Autodesk Inventor part; units mm, degrees
ref_plane "YZ Plane" through (0, 0, 0) normal (1, 0, 0) x (0, 1, 0)
ref_plane "XZ Plane" through (0, 0, 0) normal (0, 1, 0) x (-1, 0, 0)
ref_plane "XY Plane" through (0, 0, 0) normal (0, 0, 1) x (1, 0, 0)
sketch "Sketch1" plane through (0, 0, 0) normal (0, 1, 0) x (-1, 0, 0)
  line L0 (0, 0) -> (50, 0)
  line L1 (50, 0) -> (50, 460)
  line L2 (50, 460) -> (0, 460)
  line L3 (0, 460) -> (0, 0)
  circle A0 centre (25, 415) radius 12
  circle A1 centre (25, 45) radius 12
  circle A2 centre (25, 450) radius 5
  circle A3 centre (25, 10) radius 5
  line L4 (50, 280) -> (0, 280)
  line L5 (0, 280) -> (0, 180)
  line L6 (0, 180) -> (50, 180)
  line L7 (50, 180) -> (50, 280)
  circle A4 centre (25, 170) radius 5
  circle A5 centre (25, 290) radius 5
  circle A6 centre (25, 230) radius 5
  dimension "d0" = 50
  dimension "d1" = 460
  dimension "d2" = 45
  dimension "d3" = 24
  dimension "d4" = 45
  dimension "d5" = 10
  dimension "d6" = 10
  dimension "d7" = 10
  dimension "d8" = 10
  dimension "d9" = 25
  dimension "d10" = 25
  dimension "d11" = 25
  dimension "d12" = 25
  dimension "d15" = 50
  dimension "d16" = 100
  dimension "d17" = 180
  dimension "d18" = 10
  dimension "d20" = 10
  dimension "d21" = 10
  dimension "d22" = 25
  dimension "d23" = 25
  dimension "d24" = 10
  dimension "d27" = 10
  dimension "d28" = 25
  dimension "d29" = 50
extrude "Plate3" add sketch "Sketch1" along normal blind 2
fillet "Fillet3" radius 15 4 edges at (0, 1, 460) (-50, 1, 460) (0, 1, 0) (-50, 1, 0)
sketch "Sketch3" plane through (0, 2, 0) normal (0, 1, 0) x (1, 0, 0)
  circle A0 centre (-25, -105) radius 12.5
  circle A1 centre (-25, -45) radius 12
  circle A2 centre (-25, -355) radius 12.5
  circle A3 centre (-25, -415) radius 12
  point P0 (0, 0)
  dimension "d36" = 25
  dimension "d37" = 60
  dimension "d38" = 25
  dimension "d42" = 60
extrude "Extrusion1" cut sketch "Sketch3" against normal blind 10 contours A0 | A2
equation "\"d30\" = Thickness"
equation "\"BendRadius\" = Thickness"
equation "\"BendReliefWidth\" = Thickness"
equation "\"BendReliefDepth\" = 0.5 * Thickness"
equation "\"CornerReliefSize\" = 4 * Thickness"
equation "\"MinimumRemnant\" = 2 * Thickness"
equation "\"TransitionRadius\" = BendRadius"
equation "\"JacobiRadiusSize\" = BendRadius"
equation "\"GapSize\" = Thickness"
properties part number "chassisPart1"
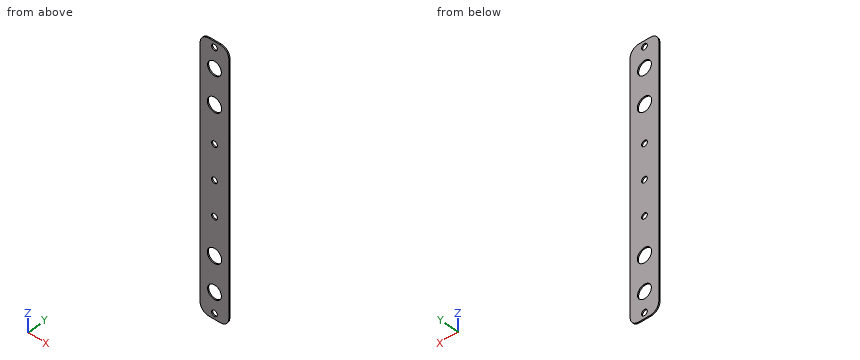
Geometry check sheet. Reference: the model listing, model coordinates, mm. Give positions to 0.01 mm unless a question says otherwise; leave off trailing zeros. Loops run counter-clockwise (first coordinate to the right, second up) from the corner with the lowest first, then second, coordinate; pieces in that order, holes last. Notation, with made-up numbers: M 64.25,-35.5 L 114.25,-35.5 A16 ccw 114.25,-21.5 Z; hole C -32,26 d4. An arc over 180 degrees is marked long. Answer as a JSON object with one key per item and string values. Group by question number.
Item 1: Material ranges on L1, parallel to Z at x = -17.5, y = 0.5; L2, parallel to Z at x = -14.5, y = 0.65; L3, parallel to X at y = 1.55, z = 105, recorded low to high.
Item 2: Sectioned sample at A-A on z = 105. Record the boundary of the cut face in (x, y), plus the area to 3 significant figures.
Item 3: Sectioned sample at C-C on z = 170. Record the boundary of the cut face in (x, y), plus the area to 3 significant figures.
Item 4: Sectioned sample at B-B on y = 1. Give the number of separate pieces and of enclosed holes in the cut face, plus the area to 3 significant figures.
Item 5: Gauge pin test, flat ends, axial feed: pin 1 (9 mm diameter, centred on x = -25, z = 450, fed in from +Y); pin 2 (1 mm diameter, centred on x = -11, y = 1, fed in from +Z). Record the tip position at first contact, or that the pin passes through.
Findings below:
{
 "1": {"L1": "0 to 35.63, 54.37 to 95, 115 to 345, 365 to 405.63, 424.37 to 460", "L2": "0.01 to 39.19, 50.81 to 98.22, 111.78 to 348.22, 361.78 to 409.19, 420.81 to 459.99", "L3": "-50 to -37.5, -12.5 to 0"},
 "2": {"outline": "M -50,0 L -37.5,0 L -37.5,2 L -50,2 Z; M -12.5,0 L 0,0 L 0,2 L -12.5,2 Z", "area": "50.0 mm2"},
 "3": {"outline": "M -50,0 L -30,0 L -30,2 L -50,2 Z; M -20,0 L 0,0 L 0,2 L -20,2 Z", "area": "80.0 mm2"},
 "4": {"separate pieces": "1", "enclosed holes": "9", "area": "20,500 mm2"},
 "5": {"pin 1": "through", "pin 2": "z = 459.59"}
}
